```python
from build123d import *

# Parameters (mm, degrees)
SKETCH_1_R      = 2.5
EXTRUDE_1_DEPTH = 100
FILLET_1_R      = 1.5


with BuildPart() as part:
    # 草图1 → 凸台-拉伸1 (new body)
    with BuildSketch(Plane.XY):
        with BuildLine():
            Line((20, 13.6), (20, 20))
            Line((20, 20), (13.6, 20))
            Line((13.6, 20), (13.6, 19.8))
            Line((13.6, 19.8), (13.2, 19.8))
            ThreePointArc((13.2, 19.8), (13.129289322, 19.770710678), (13.1, 19.7))
            Line((13.1, 19.7), (13.1, 18.3))
            ThreePointArc((13.1, 18.3), (13.129289322, 18.229289322), (13.2, 18.2))
            Line((13.2, 18.2), (15.2, 18.2))
            ThreePointArc((15.2, 18.2), (15.412132034, 18.112132034), (15.5, 17.9))
            Line((15.5, 17.9), (15.5, 16.974873734))
            ThreePointArc((15.5, 16.974873734), (15.423879533, 16.592190302), (15.207106781, 16.267766953))
            Line((15.207106781, 16.267766953), (13.132233047, 14.192893219))
            ThreePointArc((13.132233047, 14.192893219), (12.807809698, 13.976120467), (12.425126266, 13.9))
            Line((12.425126266, 13.9), (7.574873734, 13.9))
            ThreePointArc((7.574873734, 13.9), (7.192190302, 13.976120467), (6.867766953, 14.192893219))
            Line((6.867766953, 14.192893219), (4.792893219, 16.267766953))
            ThreePointArc((4.792893219, 16.267766953), (4.576120467, 16.592190302), (4.5, 16.974873734))
            Line((4.5, 16.974873734), (4.5, 17.9))
            ThreePointArc((4.5, 17.9), (4.587867966, 18.112132034), (4.8, 18.2))
            Line((4.8, 18.2), (6.8, 18.2))
            ThreePointArc((6.8, 18.2), (6.870710678, 18.229289322), (6.9, 18.3))
            Line((6.9, 18.3), (6.9, 19.7))
            ThreePointArc((6.9, 19.7), (6.870710678, 19.770710678), (6.8, 19.8))
            Line((6.8, 19.8), (6.4, 19.8))
            Line((6.4, 19.8), (6.4, 20))
            Line((6.4, 20), (0, 20))
            Line((0, 20), (0, 13.6))
            Line((0, 13.6), (0.2, 13.6))
            Line((0.2, 13.6), (0.2, 13.2))
            ThreePointArc((0.2, 13.2), (0.229289322, 13.129289322), (0.3, 13.1))
            Line((0.3, 13.1), (1.7, 13.1))
            ThreePointArc((1.7, 13.1), (1.770710678, 13.129289322), (1.8, 13.2))
            Line((1.8, 13.2), (1.8, 15.2))
            ThreePointArc((1.8, 15.2), (1.887867966, 15.412132034), (2.1, 15.5))
            Line((2.1, 15.5), (3.025126266, 15.5))
            ThreePointArc((3.025126266, 15.5), (3.407809698, 15.423879533), (3.732233047, 15.207106781))
            Line((3.732233047, 15.207106781), (5.807106781, 13.132233047))
            ThreePointArc((5.807106781, 13.132233047), (6.023879533, 12.807809698), (6.1, 12.425126266))
            Line((6.1, 12.425126266), (6.1, 7.574873734))
            ThreePointArc((6.1, 7.574873734), (6.023879533, 7.192190302), (5.807106781, 6.867766953))
            Line((5.807106781, 6.867766953), (3.732233047, 4.792893219))
            ThreePointArc((3.732233047, 4.792893219), (3.407809698, 4.576120467), (3.025126266, 4.5))
            Line((3.025126266, 4.5), (2.1, 4.5))
            ThreePointArc((2.1, 4.5), (1.887867966, 4.587867966), (1.8, 4.8))
            Line((1.8, 4.8), (1.8, 6.8))
            ThreePointArc((1.8, 6.8), (1.770710678, 6.870710678), (1.7, 6.9))
            Line((1.7, 6.9), (0.3, 6.9))
            ThreePointArc((0.3, 6.9), (0.229289322, 6.870710678), (0.2, 6.8))
            Line((0.2, 6.8), (0.2, 6.4))
            Line((0.2, 6.4), (0, 6.4))
            Line((0, 6.4), (0, 0))
            Line((0, 0), (6.4, 0))
            Line((6.4, 0), (6.4, 0.2))
            Line((6.4, 0.2), (6.8, 0.2))
            ThreePointArc((6.8, 0.2), (6.870710678, 0.229289322), (6.9, 0.3))
            Line((6.9, 0.3), (6.9, 1.7))
            ThreePointArc((6.9, 1.7), (6.870710678, 1.770710678), (6.8, 1.8))
            Line((6.8, 1.8), (4.8, 1.8))
            ThreePointArc((4.8, 1.8), (4.587867966, 1.887867966), (4.5, 2.1))
            Line((4.5, 2.1), (4.5, 3.025126266))
            ThreePointArc((4.5, 3.025126266), (4.576120467, 3.407809698), (4.792893219, 3.732233047))
            Line((4.792893219, 3.732233047), (6.867766953, 5.807106781))
            ThreePointArc((6.867766953, 5.807106781), (7.192190302, 6.023879533), (7.574873734, 6.1))
            Line((7.574873734, 6.1), (12.425126266, 6.1))
            ThreePointArc((12.425126266, 6.1), (12.807809698, 6.023879533), (13.132233047, 5.807106781))
            Line((13.132233047, 5.807106781), (15.207106781, 3.732233047))
            ThreePointArc((15.207106781, 3.732233047), (15.423879533, 3.407809698), (15.5, 3.025126266))
            Line((15.5, 3.025126266), (15.5, 2.1))
            ThreePointArc((15.5, 2.1), (15.412132034, 1.887867966), (15.2, 1.8))
            Line((15.2, 1.8), (13.2, 1.8))
            ThreePointArc((13.2, 1.8), (13.129289322, 1.770710678), (13.1, 1.7))
            Line((13.1, 1.7), (13.1, 0.3))
            ThreePointArc((13.1, 0.3), (13.129289322, 0.229289322), (13.2, 0.2))
            Line((13.2, 0.2), (13.6, 0.2))
            Line((13.6, 0.2), (13.6, 0))
            Line((13.6, 0), (20, 0))
            Line((20, 0), (20, 6.4))
            Line((20, 6.4), (19.8, 6.4))
            Line((19.8, 6.4), (19.8, 6.8))
            ThreePointArc((19.8, 6.8), (19.770710678, 6.870710678), (19.7, 6.9))
            Line((19.7, 6.9), (18.3, 6.9))
            ThreePointArc((18.3, 6.9), (18.229289322, 6.870710678), (18.2, 6.8))
            Line((18.2, 6.8), (18.2, 4.8))
            ThreePointArc((18.2, 4.8), (18.112132034, 4.587867966), (17.9, 4.5))
            Line((17.9, 4.5), (16.974873734, 4.5))
            ThreePointArc((16.974873734, 4.5), (16.592190302, 4.576120467), (16.267766953, 4.792893219))
            Line((16.267766953, 4.792893219), (14.192893219, 6.867766953))
            ThreePointArc((14.192893219, 6.867766953), (13.976120467, 7.192190302), (13.9, 7.574873734))
            Line((13.9, 7.574873734), (13.9, 12.425126266))
            ThreePointArc((13.9, 12.425126266), (13.976120467, 12.807809698), (14.192893219, 13.132233047))
            Line((14.192893219, 13.132233047), (16.267766953, 15.207106781))
            ThreePointArc((16.267766953, 15.207106781), (16.592190302, 15.423879533), (16.974873734, 15.5))
            Line((16.974873734, 15.5), (17.9, 15.5))
            ThreePointArc((17.9, 15.5), (18.112132034, 15.412132034), (18.2, 15.2))
            Line((18.2, 15.2), (18.2, 13.2))
            ThreePointArc((18.2, 13.2), (18.229289322, 13.129289322), (18.3, 13.1))
            Line((18.3, 13.1), (19.7, 13.1))
            ThreePointArc((19.7, 13.1), (19.770710678, 13.129289322), (19.8, 13.2))
            Line((19.8, 13.2), (19.8, 13.6))
            Line((19.8, 13.6), (20, 13.6))
        make_face()
        with Locations((10, 10)):
            Circle(SKETCH_1_R, mode=Mode.SUBTRACT)
    extrude(amount=EXTRUDE_1_DEPTH)

    # 圆角1
    fillet_1_edges = [part.edges().sort_by_distance(p)[0] for p in [
        (0, 0, 50),
        (0, 20, 50),
        (20, 20, 50),
        (20, 0, 50),
    ]]
    fillet(fillet_1_edges, radius=FILLET_1_R)


solid = part.part
```
Here's how the part is built. I have some questions about the finished solid (model axes, mm). A direction names the side the tool comes from. Give positions to 0.01 mm unless a question says otherwise; leave off trailing zeros. Order: outer loops, then holes, each group sorted by start corner. A loop starts at its lowest first (then second) coordinate and runs counter-clockwise, first axis right, second up. Notation, with made-up numbers: (73.5, 55) - (93.5, 55) arc R30 ccw to (93.5, 90) - close; hole circle Ø4 at (40.25, 24.5). An arc over 180 degrees is marked (long way). Answer as a JSON object with one key per item and string values. Group by question number.
Item 1: If we section it at A-A on y = 10: Please give me the cut outline in (x, z).
Item 2: For P1, Ø1.5, axis at x = 9.5, z = 63.5, coming from the +Y side; P2, Ø1.5, axis at y = 10, z = 40.5, coming from the -X side, each with a flat end and sliding along its axis, tell me the tip position at first contact or that it passes through.
Item 3: Please list where these lines run through material, in increasing order: probe 1 along X at (y, z) = (2.25, 87); probe 2 along Y at (x, z) = (10, 45.5); probe 3 along Y at (x, z) = (1.75, 51.5).
Item 4: If we mould it in two halves opening along X, with no side actions, what happens to faces 3 (the flat face through (13.9, 10, 49)), 4 (the flat face through (0, 4, 49)), 5 (the flat face through (4, 0, 49)), 6 (the flat face through (1.8, 14, 49))? For each: pulls with the +X half, pulls with the -X half, needs draft (parallel to the pull), parting line crosses it, or undercut.
Item 5: Which directions (+Z, -Z, +X, -X, +Y, -Y) give clear straight access to the entire face, cutting with the end or side of a thin tool? Please do faces 1 (the flat face through (8, 12, 100)), 2 (the flat face through (4.76, 14.18, 49.3)).
Result set:
{
 "1": {"outline": "(6.1, 0) - (7.5, 0) - (7.5, 100) - (6.1, 100) - close; (12.5, 0) - (13.9, 0) - (13.9, 100) - (12.5, 100) - close"},
 "2": {"P1": "y = 13.9", "P2": "x = 6.1"},
 "3": {"probe 1": "0 to 4.5, 15.5 to 20", "probe 2": "6.1 to 7.5, 12.5 to 13.9", "probe 3": "0 to 6.89, 13.11 to 20"},
 "4": {"face 3": "pulls with the +X half", "face 4": "pulls with the -X half", "face 5": "needs draft", "face 6": "undercut"},
 "5": {"face 1": "+Z, +X, -X, +Y, -Y", "face 2": "+Z, -Z"}
}
